Could you check a few things on this model? Use its own coordinates, in mm. A direction names the side the tool comes from. Coordinates: 2 decimals unless noted, no trailing zeros. Write each loop counter-clockwise with the first axis right and the second up, starting at its lowest first coordinate (ties: lowest second). Pieces come first, ordered by that corner, then holes.
```python
from build123d import *

# Parameters (mm, degrees)
CROQUIS1_R              = 9.525
CROQUIS1_R_2            = 3.175
SALIENTE_EXTRUIR1_DEPTH = 3.175
CROQUIS2_R              = 2.54
CORTAR_EXTRUIR1_DEPTH   = 3.175
CROQUIS3_W              = 1.5875
CROQUIS3_H              = 3.175
CORTAR_EXTRUIR2_DEPTH   = 14.430129201


with BuildPart() as part:
    # Croquis1 → Saliente-Extruir1 (new body)
    with BuildSketch(Plane.XY):
        Circle(CROQUIS1_R)
        Circle(CROQUIS1_R_2, mode=Mode.SUBTRACT)
    extrude(amount=SALIENTE_EXTRUIR1_DEPTH)

    # Croquis2 → Cortar-Extruir1 (cut)
    with BuildSketch(Plane.XY.offset(3.175)):
        with Locations((-10.16, 0)):
            Circle(CROQUIS2_R)
        with Locations((-7.184204897, 7.184204897)):
            Circle(CROQUIS2_R)
        with Locations((0, 10.16)):
            Circle(CROQUIS2_R)
        with Locations((7.184204897, 7.184204897)):
            Circle(CROQUIS2_R)
        with Locations((10.16, 0)):
            Circle(CROQUIS2_R)
        with Locations((7.184204897, -7.184204897)):
            Circle(CROQUIS2_R)
        with Locations((0, -10.16)):
            Circle(CROQUIS2_R)
        with Locations((-7.184204897, -7.184204897)):
            Circle(CROQUIS2_R)
    extrude(amount=-CORTAR_EXTRUIR1_DEPTH, mode=Mode.SUBTRACT)

    # Croquis3 → Cortar-Extruir2 (cut, through all)
    with BuildSketch(Plane(origin=(0, 0, 0), x_dir=(1, 0, 0), z_dir=(0, 1, 0))):
        with Locations((0, -1.5875)):
            Rectangle(CROQUIS3_W, CROQUIS3_H)
    extrude(amount=CORTAR_EXTRUIR2_DEPTH, mode=Mode.SUBTRACT)


solid = part.part
```
Item 1: Will these pins go through, and if not, where does the flat tip stop? pin 1 Ø1.5 at (y, z) = (-3, 1) entering from +X; pin 2 Ø1 at (y, z) = (6, 2) entering from -X.
Item 2: I want a section at A-A, the plane y = 0. List the corners of the cut face in (x, z) for me (3 decimals), then the cut area to 3 significant figures.
Item 3: I want a section at C-C, the plane x = 0. List the corners of the cut face in (y, z) for me (3 decimals).
Item 4: I want a section at B-B, the plane z = 2.7. List the corners of the cut face in (x, y) for me (3 decimals).
Item 5: Which directions (+Z, -Z, +X, -X, +Y, -Y) give clear straight access to the entire face, cutting with the end or side of a thin tool? Please do faces 1 (the cylindrical face through (-5.418, 5.358, 1.61)), 2 (the cylindrical face through (-1.75, 8.32, 1.61)).
Item 6: If I drill on line 1 along Y through (x, z) = (0, 1.2) (3 decimals); line 2 along X through (y, z) = (7.5, 2.4); line 3 along X through (y, z) = (5.25, 2.8), over which ranges is the centre line in solid material (lowest first)?
Item 7: I want a section at D-D, the plane y = 6.25. List the corners of the cut face in (x, z) for me (3 decimals), then the cut area to 3 significant figures.
Taken from the geometry:
1. pin 1: stops at x = 9.23
1. pin 2: stops at x = -5.28
2. outline: (-7.62, 0) - (-3.175, 0) - (-3.175, 3.175) - (-7.62, 3.175) - close; (3.175, 0) - (7.62, 0) - (7.62, 3.175) - (3.175, 3.175) - close
2. area: 28.2 mm2
3. outline: (-7.62, 0) - (-3.175, 0) - (-3.175, 3.175) - (-7.62, 3.175) - close
4. outline: (-9.227, -2.363) arc R9.525 ccw to (-8.195, -4.854) arc R2.54 cw to (-4.854, -8.195) arc R9.525 ccw to (-2.363, -9.227) arc R2.54 cw to (2.363, -9.227) arc R9.525 ccw to (4.854, -8.195) arc R2.54 cw to (8.195, -4.854) arc R9.525 ccw to (9.227, -2.363) arc R2.54 cw to (9.227, 2.363) arc R9.525 ccw to (8.195, 4.854) arc R2.54 cw to (4.854, 8.195) arc R9.525 ccw to (2.363, 9.227) arc R2.54 cw to (0.794, 7.747) - (0.794, 3.074) arc R3.175 cw (long way) to (-0.794, 3.074) - (-0.794, 7.747) arc R2.54 cw to (-2.363, 9.227) arc R9.525 ccw to (-4.854, 8.195) arc R2.54 cw to (-8.195, 4.854) arc R9.525 ccw to (-9.227, 2.363) arc R2.54 cw to start
5. face 1: +Z, -Z
5. face 2: +Z, -Z, +Y
6. line 1: y = -7.62 to -3.175
6. line 2: x = -4.66 to -0.79, 0.79 to 4.66
6. line 3: x = -5.54 to -0.79, 0.79 to 5.54
7. outline: (-4.822, 0) - (-0.794, 0) - (-0.794, 3.175) - (-4.822, 3.175) - close; (0.794, 0) - (4.822, 0) - (4.822, 3.175) - (0.794, 3.175) - close
7. area: 25.6 mm2
